```python
from build123d import *

# Parameters (mm, degrees)
F1_DEPTH = 25.4


with BuildPart() as f1:
    # F0 (on Right) → F1 (new body)
    with BuildSketch(Plane.YZ):
        Polygon((-34.4482409456, -28.3169634459), (-36.5716814995, -31.596750021), (-32.3062588394, -34.5458548038), align=None)
        Polygon((-34.4482409456, -28.3169634459), (-32.3062588394, -34.5458548038), (18.8768748194, -69.9337720871), (16.9203405898, -51.5107249157), (-28.9372427897, -19.8048825524), align=None)
        Polygon((18.8768748194, -69.9337720871), (-32.3062588394, -34.5458548038), (17.1237699687, -178.2885491848), align=None)
        Polygon((-40.0073602796, -12.1510252357), (-34.4482409456, -28.3169634459), (-28.9372427897, -19.8048825524), align=None)
        Polygon((-40.0073602796, -12.1510252357), (-28.9372427897, -19.8048825524), (-12.2332527089, 5.9954735336), (-87.3578041792, 104.4562384486), align=None)
        Polygon((-12.2332527089, 5.9954735336), (-28.9372427897, -19.8048825524), (16.9203405898, -51.5107249157), (14.5396798196, -29.0940326822), align=None)
        Polygon((14.5396798196, -29.0940326822), (16.9203405898, -51.5107249157), (48.0821750748, -73.0559555868), align=None)
        Polygon((7.5655095279, 36.5758985281), (-12.2332527089, 5.9954735336), (14.5396798196, -29.0940326822), align=None)
    extrude(amount=F1_DEPTH)


solid = f1.part
```
Part model, mm, in its own coordinate system. A direction names the side the tool comes from. Coordinates: 2 decimals unless noted, no trailing zeros. Write each loop counter-clockwise with the first axis right and the second up, starting at its lowest first coordinate (ties: lowest second). Pieces come first, ordered by that corner, then holes.
Item 1: Slice it at B-B (x = 15). Write the cut outline in (y, z), and give its area (3 significant figures).
Item 2: Slice it at C-C (y = -7). Write the cut outline in (x, z).
Item 3: Which spindle directions (+Z, -Z, +X, -X, +Y, -Y) get a long thin tool onto all of the face, cutting with end or side? Do faces 1 (the face through (12.522, 17.912, -60.851)), 2 (the face through (12.52, -49.27, 54.54)), 3 (the face through (0, -15, -26)). Say none if no direction does.
Item 4: Slice it at A-A (z = 20.5). Write the cut outline in (x, y).
Item 5: Slice it at D-D (z = -63). Write the cut outline in (x, y).
Item 6: Pin check, flat tips, straight feed: pin 1 (10 mm diameter, centred on x = 19, z = 68.5, fed in from -Y); pin 2 (1.5 mm diameter, centred on x = 16, y = 32, fed in from +Z); pin 3 (12 mm diameter, centred on x = 6, y = -23.5, fed in from +Z). Stop position of each tip, or through.
Item 7: Probe line 1 (Y direction, x = 15, z = 24); line 2 (Y direction, x = 3.5, z = 15); line 3 (Y direction, x = 20.5, z = 91). List the from-to ranges inside material, lowest first.
Item 8: Mould opens along Y. For faces 4 (the face through (12.522, -37.267, -20.121)), 5 (the face through (12.522, -2.195, 21.5)), 6 (the face through (25.4, -15, -26)) say: released by +Y, released by -Y, zero draft, split by the parting line, or undercut.
Results found:
1. outline: (-87.36, 104.46) - (-40.01, -12.15) - (-34.45, -28.32) - (-36.57, -31.6) - (-32.31, -34.55) - (17.12, -178.29) - (18.88, -69.93) - (16.92, -51.51) - (48.08, -73.06) - (14.54, -29.09) - (7.57, 36.58) - (-12.23, 6) - close
1. area: 8,190 mm2
2. outline: (0, -108.14) - (25.4, -108.14) - (25.4, 14.08) - (0, 14.08) - close
3. face 1: +X, -X
3. face 2: +Z, +X, -X
3. face 3: +Z, -Z, -X, +Y, -Y
4. outline: (0, -53.27) - (25.4, -53.27) - (25.4, -23.3) - (0, -23.3) - close; (0, -2.84) - (25.4, -2.84) - (25.4, 9.27) - (0, 9.27) - close
5. outline: (0, -22.52) - (25.4, -22.52) - (25.4, 18.14) - (0, 18.14) - close; (0, 33.54) - (25.4, 33.54) - (25.4, 40.41) - (0, 40.41) - close
6. pin 1: stops at y = -74.79
6. pin 2: stops at z = -51
6. pin 3: stops at z = 28.63
7. line 1: y = -54.69 to -25.97, -0.58 to 8.9
7. line 2: y = -51.03 to -19.1, -6.4 to 9.86
7. line 3: y = -81.89 to -77.09
8. face 4: released by -Y
8. face 5: undercut
8. face 6: zero draft
